Verification items for the finished model (mm, model axes). A direction names the side the tool comes from. Coordinates: 2 decimals unless noted, no trailing zeros. Loops run counter-clockwise (first coordinate to the right, second up) from the corner with the lowest first, then second, coordinate; pieces in that order, holes last.
Q1. Material ranges on probe 1 along Z at (x, y) = (136.5, 123.5); probe 2 along Y at (x, z) = (160.5, 0); probe 3 along Y at (x, z) = (160, 0), recorded low to high.
Q2. Sectioned sample at C-C (x = -40). Enter the section's corners in (y, z), then the cut area to 3 significant figures.
Q3. Access from +Z, -Z, +X, -X, +Y, -Y to the whole of each face (thin tool, end or side, straight path). Record for faces 4 (the face through (150, 69, -76)), 5 (the face through (126, 73, 83.75)), 6 (the face through (137, 147.5, -1)), 7 (the face through (126, 73, -83.75)), 8 (the face through (158.872, 10.542, -8.299)).
Q4. Mould release check, pull along Z, two halves, no side actions. Record for faces 1 (the face through (150, 75, 1)), 2 (the face through (150, 74, 76)), 3 (the face through (166.405, 9.922, -8.38)): +Z half, -Z half, draft (parallel to the pull), parting line (faces both ways), or undercut.
Q5. Go/stop test with flat-tipped pins: P1, Ø4, axis at y = 22, z = 96.5, coming from the +X side; P2, Ø1, axis at y = 88, z = -85.5, coming from the +X side; P3, Ø8, axis at y = 121.5, z = 77, coming from the -X side. Record where each tip stops, or that it passes through.
Q6. Sectioned sample at B-B (z = 79). Enter the section's corners in (x, y).
Q7. Sectioned sample at D-D (z = 115.5). Enter the section's corners in (x, y).
```python
from build123d import *

# Parameters (mm, degrees)
SKETCH1_R           = 132.8125
BOSS_EXTRUDE1_DEPTH = 147.5
SKETCH2_W           = 167.5
SKETCH2_H           = 147.5
BOSS_EXTRUDE2_DEPTH = 150
SKETCH5_R           = 132.8125
BOSS_EXTRUDE3_DEPTH = 50


with BuildPart() as part:
    # Sketch1 → Boss-Extrude1 (new body)
    with BuildSketch(Plane(origin=(0, 0, 0), x_dir=(1, 0, 0), z_dir=(0, 1, 0))):
        with Locations(Location((0, 0, 0), (0, 0, 270))):
            Circle(SKETCH1_R)
    extrude(amount=BOSS_EXTRUDE1_DEPTH)

    # Sketch2 → Boss-Extrude2 (add)
    with BuildSketch(Plane(origin=(0, 0, 0), x_dir=(0, 0, -1), z_dir=(1, 0, 0))):
        with Locations((0, 73.75)):
            Rectangle(SKETCH2_W, SKETCH2_H)
    extrude(amount=BOSS_EXTRUDE2_DEPTH)

    # Sketch4 → Revolve1 (revolve)
    with BuildSketch(Plane.XY, mode=Mode.PRIVATE) as revolve1_sk:
        Polygon((150, 0), (150, 10), (167.5, 10), align=None)
    revolve(revolve1_sk.sketch.rotate(Axis((150, 73.75, 0), (1, 0, 0)), 270), axis=Axis((150, 73.75, 0), (1, 0, 0)))

    # Sketch5 → Boss-Extrude3 (add)
    with BuildSketch(Plane(origin=(0, 147.5, 0), x_dir=(1, 0, 0), z_dir=(0, 1, 0))):
        with Locations(Location((0, 0, 0), (0, 0, 39.093534815))):
            Circle(SKETCH5_R)
    extrude(amount=BOSS_EXTRUDE3_DEPTH)


solid = part.part
```
Geometry check:
1. probe 1: z = -83.75 to 83.75
1. probe 2: y = 6 to 10, 137.5 to 141.5
1. probe 3: y = 5.71 to 10, 137.5 to 141.79
2. outline: (0, -126.65) - (197.5, -126.65) - (197.5, 126.65) - (0, 126.65) - close
2. area: 50,000 mm2
3. face 4: -Z, +X
3. face 5: +Z, +X, +Y, -Y
3. face 6: +X, +Y
3. face 7: -Z, +X, +Y, -Y
3. face 8: +X
4. face 1: undercut
4. face 2: draft
4. face 3: parting line
5. P1: stops at x = 93.32
5. P2: stops at x = 102.05
5. P3: stops at x = -110.95
6. outline: (-106.76, 0) - (150, 0) - (150, 147.5) - (106.76, 147.5) - (106.76, 197.5) - (-106.76, 197.5) - close
7. outline: (-65.57, 0) - (65.57, 0) - (65.57, 197.5) - (-65.57, 197.5) - close
